Autodesk Fusion 360 part; units mm, degrees
sketch "Sketch1" plane through (0, 0, 0) normal (0, 0, 1) x (1, 0, 0)
  circle A0 centre (0, 0) radius 4
  dimension "d1" = 8
extrude "Extrude1" add sketch "Sketch1" along normal blind 2.5
fillet "Fillet1" radius 0.2 1 edges at (-3.7293, -1.4465, 2.5)
fillet "Fillet2" radius 0.2 1 edges at (-3.7293, -1.4465, 0)
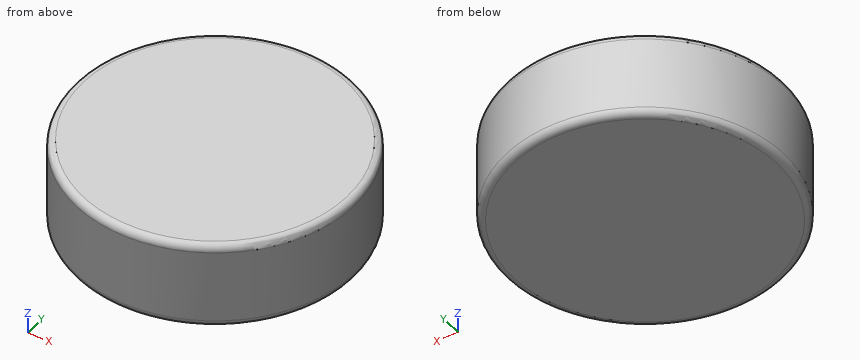
CAD build for the part. Positions are in the model's coordinates, mm. Give positions to 0.01 mm unless a question says otherwise; leave off trailing zeros. Loops run counter-clockwise (first coordinate to the right, second up) from the corner with the lowest first, then second, coordinate; pieces in that order, holes last. Notation, with made-up numbers: (80.5, 21) -> (99.5, 21) arc R26 ccw to (99.5, 39) -> close; hole circle Ø2 at (-12, -36.5). An arc over 180 degrees is marked (long way). Use a Markdown table: item, result.
1. Slice it at A-A (z = 1.75). List the corners of the cut face in (x, y).
Check result:
| item | result |
|---|---|
| outline | circle Ø8 at (0, 0) |
2. Flat gauge pins, fed straight in: pin 1 (2 mm diameter, centred on x = -2, y = -1.5, fed in from -Z); pin 2 (1.5 mm diameter, centred on y = -2, z = 1.5, fed in from +X); pin 3 (1.5 mm diameter, centred on y = -2.5, z = 1, fed in from -X); pin 4 (1.5 mm diameter, centred on x = -2.5, z = 1, fed in from -Y). Where does each tip first touch, or does it go through?
Check result:
| item | result |
|---|---|
| pin 1 | stops at z = 0 |
| pin 2 | stops at x = 3.8 |
| pin 3 | stops at x = -3.6 |
| pin 4 | stops at y = -3.6 |
3. Wall check: L1, parallel to X at y = 1.25, z = 0.65; L2, parallel to X at y = -1.5, z = 0.2. Give the ranges that are in metal, low to high. Write a range as [from, to].
Check result:
| item | result |
|---|---|
| L1 | x = [-3.8, 3.8] |
| L2 | x = [-3.71, 3.71] |
